```python
from build123d import *

# Parameters (mm, degrees)
SKETCH1_5_R             = 1.1938
CUT_EXTRUDE1_DEPTH      = 12.8999
CUT_EXTRUDE1_DEPTH_BACK = 12.8999
SKETCH2_R               = 1.1938
CUT_EXTRUDE2_DEPTH      = 17.6624001


with BuildPart() as part:
    # Sketch1 → Revolve1 (revolve)
    with BuildSketch(Plane(origin=(0, 0, 0), x_dir=(0, 0, -1), z_dir=(1, 0, 0))):
        Polygon((3.9243, 0), (2.3876, 0), (2.3876, 16.6624), (5.3975, 16.6624), (5.3975, 3.175), (11.8999, 3.175), (11.8999, 1.5875), (3.9243, 1.5875), align=None)
    revolve(axis=Axis((0, 0, 0), (0, 1, 0)))

    # Sketch1_5 → Cut-Extrude1 (cut, two sides)
    with BuildSketch(Plane(origin=(0, 0, 0), x_dir=(0, 0, -1), z_dir=(1, 0, 0))) as cut_extrude1_sk:
        with Locations((0, 12.7)):
            Circle(SKETCH1_5_R)
    extrude(amount=CUT_EXTRUDE1_DEPTH, mode=Mode.SUBTRACT)
    extrude(cut_extrude1_sk.sketch, amount=-CUT_EXTRUDE1_DEPTH_BACK, mode=Mode.SUBTRACT)

    # Sketch2 → Cut-Extrude2 (cut, through all)
    with BuildSketch(Plane(origin=(0, 0, 0), x_dir=(1, 0, 0), z_dir=(0, 1, 0))):
        with Locations(Location((-8.3312, 0, 0), (0, 0, 90))):  # turned: the seam where the file's is
            Circle(SKETCH2_R)
        with Locations(Location((0, 8.3312, 0), (0, 0, 90))):  # turned: the seam where the file's is
            Circle(SKETCH2_R)
        with Locations(Location((0, -8.3312, 0), (0, 0, 90))):  # turned: the seam where the file's is
            Circle(SKETCH2_R)
        with Locations(Location((8.3312, 0, 0), (0, 0, 90))):  # turned: the seam where the file's is
            Circle(SKETCH2_R)
    extrude(amount=CUT_EXTRUDE2_DEPTH, mode=Mode.SUBTRACT)


solid = part.part
```
The model under review builds one solid part; all positions refer to its coordinate system, in mm. A direction names the side the tool comes from. Round coordinates to 2 decimals unless told otherwise and drop trailing zeros. Write each loop counter-clockwise with the first axis right and the second up, starting at its lowest first coordinate (ties: lowest second). Pieces come first, ordered by that corner, then holes.
(1) We need section B-B on x = 0. Give the boundary of the cut face in (y, z) (1 decimal), and give its area (3 significant figures).
(2) Wall thickness on L1, parallel to X at y = 2.35, z = 0 (3 decimals); L2, parallel to X at y = 2.25, z = 0.25; L3, parallel to Y at x = -5.25, z = 8.5 (1 decimal): over which ranges is each line inside the solid? List them lowest first.
(3) We need section C-C on x = 8.75. Give the boundary of the cut face in (y, z) (1 decimal).
(4) We need section A-A on z = 0. Give the number of separate pieces and of enclosed holes in the cut face, and give its area (3 significant figures).
(5) Machinability: for faces 1 (the cylindrical face through (-1.62, 9.82, -5.15)), 2 (the cylindrical face through (-1.179, 0.783, -3.743)), 3 (the cylindrical face through (3.711, 12.752, 1.193)), which of the approach directions +Z, -Z, +X, -X, +Y, -Y give a long, thin tool a straight path to every point of the face, cutting with its end or side? Answer none if there is none.
(6) Mouldability with a two-part tool opening along X and no side actions: class faces 4 (the flat face through (5.1, 3.175, 2.5)), 5 (the cylindrical face through (-0.717, 8.448, -2.277)), 6 (the cylindrical face through (7.241, 2.37, 9.443)) as +X half, -X half, draft (parallel to the pull), parting line (faces both ways), or undercut.
(7) Insertion check: pin 1 (6 mm diameter, centred on y = 6.5, z = 4, fed in from +X); pin 2 (4 mm diameter, centred on x = -5, y = 15, fed in from -Z); pin 3 (1.4 mm diameter, centred on y = 12.7, z = 0, fed in from -X); pin 4 (6 mm diameter, centred on x = -5, y = 10.5, fed in from -Z). Each pin has a flat end and moves straight along its axis. Give the tip position at first contact, or say it passes through.
(8) We need section D-D on z = 8.5. Give the boundary of the cut face in (x, y) (1 decimal), and give its area (3 significant figures).
Findings below:
1. outline: (0, -3.9) - (1.6, -3.9) - (1.6, -7.1) - (3.2, -7.1) - (3.2, -5.4) - (16.7, -5.4) - (16.7, -2.4) - (0, -2.4) - close; (0, 2.4) - (16.7, 2.4) - (16.7, 5.4) - (3.2, 5.4) - (3.2, 7.1) - (1.6, 7.1) - (1.6, 3.9) - (0, 3.9) - close; (1.6, -11.9) - (3.2, -11.9) - (3.2, -9.5) - (1.6, -9.5) - close; (1.6, 9.5) - (3.2, 9.5) - (3.2, 11.9) - (1.6, 11.9) - close
1. area: 109 mm2
2. L1: x = -11.9 to -9.525, -7.137 to -2.388, 2.388 to 7.137, 9.525 to 11.9
2. L2: x = -11.9 to -9.5, -7.16 to -2.37, 2.37 to 7.16, 9.5 to 11.9
2. L3: y = 1.6 to 3.2
3. outline: (1.6, -8.1) - (3.2, -8.1) - (3.2, -1.1) - (1.6, -1.1) - close; (1.6, 1.1) - (3.2, 1.1) - (3.2, 8.1) - (1.6, 8.1) - close
4. separate pieces: 6
4. enclosed holes: 0
4. area: 94.3 mm2
5. face 1: +Y
5. face 2: -Y
5. face 3: +X, -X
6. face 4: draft
6. face 5: undercut
6. face 6: parting line
7. pin 1: stops at x = 5.3
7. pin 2: stops at z = -4.49
7. pin 3: passes through
7. pin 4: stops at z = -5.01
8. outline: (-8.3, 1.6) - (-1.2, 1.6) - (-1.2, 3.2) - (-8.3, 3.2) - close; (1.2, 1.6) - (8.3, 1.6) - (8.3, 3.2) - (1.2, 3.2) - close
8. area: 22.7 mm2
